Part model, mm, in its own coordinate system. A direction names the side the tool comes from. Round coordinates to 2 decimals unless told otherwise and drop trailing zeros. Write each loop counter-clockwise with the first axis right and the second up, starting at its lowest first coordinate (ties: lowest second). Pieces come first, ordered by that corner, then holes. Notation, with made-up numbers: M -21.5,87 L -1.5,87 A21 cw -1.5,94 Z; hole C -36.5,89.25 d3. An arc over 180 degrees is marked long. Use a Markdown table: item, result. Add a question column.
1) Drop flat-ended pins along their axis: P1, Ø1, axis at y = 7, z = 10, coming from the +X side; P2, Ø1.5, axis at x = -6.5, z = 9, coming from the +Y side; P3, Ø1.5, axis at y = 5.5, z = 13, coming from the -X side; P4, Ø2, axis at x = -8, y = 2.5, coming from the -Z side. Give the stop position or say it passes through.
2) Slice it at A-A on x = -10.25. Write the cut outline in (y, z).
3) Slice it at C-C on z = 15. Write the cut outline in (x, y).
4) Wall check: probe 1 along Y at (x, z) = (-5.75, 12.25); probe 2 along X at (y, z) = (-5.25, 10.75); probe 3 along X at (y, z) = (2.75, 14.5). Give the ranges that are in metal, low to high.
5) Slice it at B-B on y = 1. Write the cut outline in (x, z).
6) Which spindle directions (+Z, -Z, +X, -X, +Y, -Y) get a long thin tool onto all of the face, cutting with end or side? Do faces 1 (the face through (-9.393, -5.009, 11.531)), 2 (the face through (-9.393, 10.089, 11.073)), 3 (the face through (-10, 15.24, 11)). Say none if no direction does.
7) Slice it at D-D on x = -14. Write the cut outline in (y, z).
```python
from build123d import *

# Parameters (mm, degrees)
SKETCH1_R           = 5.08
BOSS_EXTRUDE2_DEPTH = 5.08
SKETCH2_R           = 0.762
BOSS_EXTRUDE3_DEPTH = 10.16
SKETCH3_R           = 0.762
BOSS_EXTRUDE4_DEPTH = 10.16


with BuildPart() as part:
    # Sketch1 → Boss-Extrude2 (new body)
    with BuildSketch(Plane(origin=(0, 0, 0), x_dir=(1, 0, 0), z_dir=(0, 1, 0))):
        with Locations((-10.119861789, -11.302088634)):
            Circle(SKETCH1_R)
    extrude(amount=BOSS_EXTRUDE2_DEPTH)

    # Sketch2 → Boss-Extrude3 (add)
    with BuildSketch(Plane(origin=(0, 5.08, 0), x_dir=(1, 0, 0), z_dir=(0, 1, 0))):
        with Locations((-10.119861789, -11.302088634)):
            Circle(SKETCH2_R)
    extrude(amount=BOSS_EXTRUDE3_DEPTH)

    # Sketch3 → Boss-Extrude4 (add)
    with BuildSketch(Plane.XZ):
        with Locations((-10.119861789, 11.302088634)):
            Circle(SKETCH3_R)
    extrude(amount=BOSS_EXTRUDE4_DEPTH)


solid = part.part
```
Entries:
| question | item | result |
|---|---|---|
| 1 | P1 | passes through |
| 1 | P2 | stops at y = 5.08 |
| 1 | P3 | stops at x = -15.08 |
| 1 | P4 | stops at z = 6.35 |
| 2 | outline | M -10.16,10.55 L 0,10.55 L 0,6.22 L 5.08,6.22 L 5.08,10.55 L 15.24,10.55 L 15.24,12.05 L 5.08,12.05 L 5.08,16.38 L 0,16.38 L 0,12.05 L -10.16,12.05 Z |
| 3 | outline | M -13.6,0 L -6.64,0 L -6.64,5.08 L -13.6,5.08 Z |
| 4 | probe 1 | y = 0 to 5.08 |
| 4 | probe 2 | x = -10.65 to -9.59 |
| 4 | probe 3 | x = -14.07 to -6.17 |
| 5 | outline | C -10.12,11.3 d10.16 |
| 6 | face 1 | -Y |
| 6 | face 2 | +Y |
| 6 | face 3 | +Z, -Z, +X, -X, +Y |
| 7 | outline | M 0,8.02 L 5.08,8.02 L 5.08,14.58 L 0,14.58 Z |
